Can you work these out from the model? Positions are in its coordinate system, mm. A direction names the side the tool comes from. Give positions to 0.01 mm unless a question says otherwise; leave off trailing zeros. Order: outer loops, then holes, each group sorted by start corner. A loop starts at its lowest first (then second) coordinate and runs counter-clockwise, first axis right, second up. Notation, with made-up numbers: (11, -29.5) -> (59, -29.5) arc R11 ccw to (59, -16.5) -> close; hole circle Ø10 at (37, -1.75). An arc over 180 degrees is marked (long way). Answer as CSV lines item,"result".
```python
from build123d import *

# Parameters (mm, degrees)
BOSS_EXTRUDE1_DEPTH      = 8.65
BOSS_EXTRUDE1_DEPTH_BACK = 8.65
SKETCH2_W                = 26.6
SKETCH2_H                = 11.5
CUT_EXTRUDE1_DEPTH       = 23.566402017
SKETCH4_W                = 5.8
SKETCH4_H                = 8.8
CUT_EXTRUDE2_DEPTH       = 20.594961087
SKETCH5_W                = 1.5
SKETCH5_H                = 4.03
CUT_EXTRUDE3_DEPTH       = 3
CUT_EXTRUDE4_DEPTH       = 1.4
CUT_EXTRUDE5_START       = -5.1792
CUT_EXTRUDE5_DEPTH       = 4
FILLET3_START            = -7
FILLET3_DEPTH            = 6.429203884
FILLET4_START            = -7
FILLET4_DEPTH            = 6.429203884
CUT_EXTRUDE6_DEPTH       = 23.566402102
FILLET5_R                = 1
SKETCH12_W               = 12
SKETCH12_H               = 1.4
SKETCH12_H_2             = 0.7
CUT_EXTRUDE7_DEPTH       = 10


with BuildPart() as part:
    # Sketch2 → Boss-Extrude1 (new, two sides: drawn at the far end of the back side and taken through both)
    with BuildSketch(Plane.XY.offset(-BOSS_EXTRUDE1_DEPTH_BACK)):
        Rectangle(SKETCH2_W, SKETCH2_H)
    extrude(amount=BOSS_EXTRUDE1_DEPTH + BOSS_EXTRUDE1_DEPTH_BACK)

    # Sketch3 → Cut-Extrude1 (cut, through all)
    with BuildSketch(Plane.XY.offset(8.65)):
        with BuildLine():
            Line((-7.5, 5.75), (-7.5, -0.570796116))
            ThreePointArc((-7.5, -0.570796116), (-8.232233047, -2.338563069), (-10, -3.070796116))
            Line((-10, -3.070796116), (-13.3, -3.070796116))
            Line((-13.3, -3.070796116), (-13.3, 5.75))
            Line((-13.3, 5.75), (-7.5, 5.75))
        make_face()
        with BuildLine():
            Line((7.5, 5.75), (7.5, -0.570796116))
            ThreePointArc((7.5, -0.570796116), (8.232233047, -2.338563069), (10, -3.070796116))
            Line((10, -3.070796116), (13.3, -3.070796116))
            Line((13.3, -3.070796116), (13.3, 5.75))
            Line((13.3, 5.75), (7.5, 5.75))
        make_face()
    extrude(amount=-CUT_EXTRUDE1_DEPTH, mode=Mode.SUBTRACT)

    # Sketch4 → Cut-Extrude2 (cut, through all)
    with BuildSketch(Plane.XZ.offset(5.75)):
        with Locations((-10.4, -4.25)):
            Rectangle(SKETCH4_W, SKETCH4_H)
        with Locations((10.4, -4.25)):
            Rectangle(SKETCH4_W, SKETCH4_H)
    extrude(amount=-CUT_EXTRUDE2_DEPTH, mode=Mode.SUBTRACT)

    # Sketch5 → Cut-Extrude3 (cut)
    with BuildSketch(Plane.XZ.offset(5.75)):
        with Locations((-6.75, 4.27363419)):
            Rectangle(SKETCH5_W, SKETCH5_H)
    cut_extrude3 = extrude(amount=-CUT_EXTRUDE3_DEPTH, mode=Mode.SUBTRACT)

    # Sketch5<3> → Cut-Extrude4 (cut)
    with BuildSketch(Plane.XZ.offset(5.75)):
        with BuildLine():
            ThreePointArc((-9.05, 3.04359822), (-10.2, 4.19359822), (-9.05, 5.34359822))
            Line((-9.05, 5.34359822), (-7.5, 5.34359822))
            Line((-7.5, 5.34359822), (-7.5, 3.04359822))
            Line((-7.5, 3.04359822), (-9.05, 3.04359822))
        make_face()
    cut_extrude4 = extrude(amount=-CUT_EXTRUDE4_DEPTH, mode=Mode.SUBTRACT)

    # Sketch8 → Cut-Extrude5 (cut)
    with BuildSketch(Plane.XZ.offset(5.75).offset(CUT_EXTRUDE5_START)):
        Polygon((-11.329479063, 5.816116205), (-11.329479063, 2.651116205), (-9.259735425, 1.596272871), (-7.5, 2.651116205), (-7.5, 5.816116205), (-9.259735425, 6.763868097), align=None)
    cut_extrude5 = extrude(amount=CUT_EXTRUDE5_DEPTH, mode=Mode.SUBTRACT)

    # Fillet3: read off the stored shape, not the designer's step
    # Fillet3 outline → Fillet3 (cut)
    with BuildSketch(Plane(origin=(0, 0, 0), x_dir=(1, 0, 0), z_dir=(0, 1, 0)).offset(FILLET3_START)):
        with BuildLine():
            Line((-13.3, -8.65), (-9.05, -8.65))
            ThreePointArc((-9.05, -8.65), (-12.05520382, -7.40520382), (-13.3, -4.4))
            Line((-13.3, -4.4), (-13.3, -8.65))
        make_face()
        with BuildLine():
            Line((-13.3, -0.15), (-13.3, -4.4))
            ThreePointArc((-13.3, -4.4), (-12.05520382, -1.39479618), (-9.05, -0.15))
            Line((-9.05, -0.15), (-13.3, -0.15))
        make_face()
    extrude(amount=FILLET3_DEPTH, mode=Mode.SUBTRACT)

    # Mirror4: Cut-Extrude3, Cut-Extrude4, Cut-Extrude5 across plane
    add(cut_extrude3.mirror(Plane(origin=(0, 0, 0), x_dir=(0, 0, 1), z_dir=(1, 0, 0))), mode=Mode.SUBTRACT)
    add(cut_extrude4.mirror(Plane(origin=(0, 0, 0), x_dir=(0, 0, 1), z_dir=(1, 0, 0))), mode=Mode.SUBTRACT)
    add(cut_extrude5.mirror(Plane(origin=(0, 0, 0), x_dir=(0, 0, 1), z_dir=(1, 0, 0))), mode=Mode.SUBTRACT)

    # Fillet4: read off the stored shape, not the designer's step
    # Fillet4 outline → Fillet4 (cut)
    with BuildSketch(Plane(origin=(0, 0, 0), x_dir=(1, 0, 0), z_dir=(0, 1, 0)).offset(FILLET4_START)):
        with BuildLine():
            Line((13.3, -0.15), (9.05, -0.15))
            ThreePointArc((9.05, -0.15), (12.05520382, -1.39479618), (13.3, -4.4))
            Line((13.3, -4.4), (13.3, -0.15))
        make_face()
        with BuildLine():
            Line((13.3, -8.65), (13.3, -4.4))
            ThreePointArc((13.3, -4.4), (12.05520382, -7.40520382), (9.049999999, -8.65))
            Line((9.049999999, -8.65), (13.3, -8.65))
        make_face()
    extrude(amount=FILLET4_DEPTH, mode=Mode.SUBTRACT)

    # Sketch10 → Cut-Extrude6 (cut, through all)
    with BuildSketch(Plane.XY.offset(8.65)):
        with BuildLine():
            Line((-6, -5.75), (6, -5.75))
            Line((6, -5.75), (6, -0.75))
            add(Edge.make_bspline(
                [(6, -0.75), (6, 1.34228193), (5.397693539, 3.219717328), (3.331465755, 4.25)],
                knots=[0, 0, 0, 0, 1, 1, 1, 1], degree=3))
            Line((3.331465755, 4.25), (3.297244701, 4.25))
            Line((3.297244701, 4.25), (-3.331465755, 4.25))
            add(Edge.make_bspline(
                [(-6, -0.75), (-6, 1.34228193), (-5.397693539, 3.219717328), (-3.331465755, 4.25)],
                knots=[0, 0, 0, 0, 1, 1, 1, 1], degree=3))
            Line((-6, -0.75), (-6, -5.75))
        make_face()
    extrude(amount=-CUT_EXTRUDE6_DEPTH, mode=Mode.SUBTRACT)

    # Fillet5
    fillet5_edges = [part.edges().sort_by_distance(p)[0] for p in [
        (-7.5, 5.75, 0),
        (7.5, 5.75, 0),
    ]]
    fillet(fillet5_edges, radius=FILLET5_R)

    # Sketch12 → Cut-Extrude7 (cut)
    with BuildSketch(Plane.XZ.offset(5.75)):
        with Locations((0, -7.95)):
            Rectangle(SKETCH12_W, SKETCH12_H)
        with Locations((0, 0.7)):
            Rectangle(SKETCH12_W, SKETCH12_H_2)
        with Locations((0, 4.2)):
            Rectangle(SKETCH12_W, SKETCH12_H_2)
    extrude(amount=-CUT_EXTRUDE7_DEPTH, mode=Mode.SUBTRACT)


solid = part.part
```
Item 1: Please list where these lines run through material, in increasing order: line 1 along Z through (x, y) = (-9, -5); line 2 along X through (y, z) = (-1.75, -2.75); line 3 along Y through (x, z) = (-10.5, 5.25).
Numbers:
line 1,"z = 0.15 to 3.04, 5.34 to 8.65"
line 2,"x = -7.5 to -6, 6 to 7.5"
line 3,"y = -5.75 to -4.57"
Item 2: Imagine slicing it at B-B, the plane x = 0.25. Please give me the cut outline in (y, z), then the cut area to 4 significant figures.
Numbers:
outline,"(4.25, -8.65) -> (5.75, -8.65) -> (5.75, 8.65) -> (4.25, 8.65) -> close"
area,"25.95 mm²"
Item 3: We'd pull the mould along Z, two halves only. Please class faces 1 (the flat face through (-5.3, 3.2, 1.05)), 2 (the flat face through (7.5, 1, -2)), 3 (the flat face through (-1, 5, -8.65)), 4 (the flat face through (7, -4, 6.289)): released by +Z, released by -Z, zero draft, split by the parting line, or undercut.
Numbers:
face 1,"undercut"
face 2,"zero draft"
face 3,"released by -Z"
face 4,"undercut"
Item 4: For pin 1 (0.5 mm diameter, centred on y = -4, z = 6, fed in from +X); pin 2 (9.5 mm diameter, centred on x = 3, z = -3.5, fed in from -Y); pin 3 (0.8 mm diameter, centred on x = -7, z = 4, fed in from -Y); pin 4 (1.3 mm diameter, centred on x = 8.5, y = -5, fed in from -Z), each with a flat end and sliding along its axis, tell me the tip position at first contact or that it passes through.
Numbers:
pin 1,"stops at x = 13.08"
pin 2,"stops at y = -5.75"
pin 3,"stops at y = -2.75"
pin 4,"stops at z = 0.15"
Item 5: Imagine slicing it at A-A, the plane y = -5. Please give me the cut outline in (x, z), then the cut area to 3 significant figures.
Numbers:
outline,"(-9.05, 0.15) -> (-7.5, 0.15) -> (-7.5, -8.65) -> (-6, -8.65) -> (-6, 2.26) -> (-7.5, 2.26) -> (-7.5, 3.04) -> (-9.05, 3.04) arc R1.15 cw to (-9.05, 5.34) -> (-7.5, 5.34) -> (-7.5, 6.29) -> (-6, 6.29) -> (-6, 8.65) -> (-9.05, 8.65) arc R4.25 ccw to start; (6, -8.65) -> (7.5, -8.65) -> (7.5, 0.15) -> (9.05, 0.15) arc R4.25 ccw to (9.05, 8.65) -> (6, 8.65) -> (6, 6.29) -> (7.5, 6.29) -> (7.5, 5.34) -> (9.05, 5.34) arc R1.15 cw to (9.05, 3.04) -> (7.5, 3.04) -> (7.5, 2.26) -> (6, 2.26) -> close"
area,"112 mm²"
Item 6: For faces 5 (the flat face through (7.5, -2, 4)), 6 (the flat face through (-5.3, 3.2, 3.85)), 7 (the flat face through (-8.172, -3.432, 6.178)), which set-ups out of +Z, -Z, +X, -X, +Y, -Y let a thin tool reach every point of the face, with its end or its side?
Numbers:
face 5,"+X, +Y"
face 6,"-Y"
face 7,"+Y"
